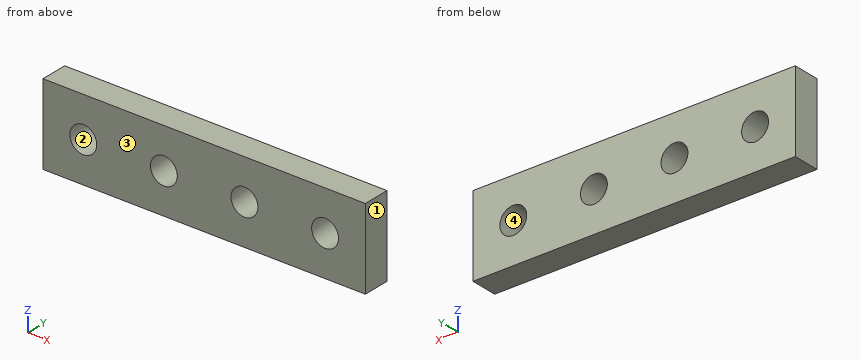
```python
from build123d import *

# Parameters (mm, degrees)
SKETCH1_W            = 120
SKETCH1_H            = 30
BOSS_EXTRUDE1_DEPTH  = 10
SKETCH2_R            = 5
CUT_EXTRUDE1_DEPTH   = 11
LPATTERN1_COUNT      = 4
LPATTERN1_PITCH      = 30
LPATTERN1_COUNT_DIR2 = 4
LPATTERN1_PITCH_DIR2 = 30


with BuildPart() as part:
    # Sketch1 → Boss-Extrude1 (new body)
    with BuildSketch(Plane(origin=(0, 0, 0), x_dir=(1, 0, 0), z_dir=(0, 1, 0))):
        with Locations((60, 15)):
            Rectangle(SKETCH1_W, SKETCH1_H)
    extrude(amount=BOSS_EXTRUDE1_DEPTH)

    # Sketch2 → Cut-Extrude1 (cut, through all)
    with BuildSketch(Plane(origin=(0, 10, 0), x_dir=(1, 0, 0), z_dir=(0, 1, 0))):
        with Locations((15, 15)):
            Circle(SKETCH2_R)
    cut_extrude1 = extrude(amount=-CUT_EXTRUDE1_DEPTH, mode=Mode.SUBTRACT)

    # LPattern1: Cut-Extrude1 4 × 4
    with Locations(*[(i * LPATTERN1_PITCH, 0, j * LPATTERN1_PITCH_DIR2) for i in range(LPATTERN1_COUNT) for j in range(LPATTERN1_COUNT_DIR2) if (i, j) != (0, 0)]):
        add(cut_extrude1, mode=Mode.SUBTRACT)


solid = part.part
```
CAD build for the part. Positions are in the model's coordinates, mm. Face numbers are marked on the shaded views. Coordinates: 2 decimals unless noted, no trailing zeros. Order: outer loops, then holes, each group sorted by start corner. A loop starts at its lowest first (then second) coordinate and runs counter-clockwise, first axis right, second up. Notation, with made-up numbers: (0, 66) - (14, 66) arc R23 cw to (14, 99) - close; hole circle Ø4 at (87.5, 23). An arc over 180 degrees is marked (long way). Use a Markdown table: item, result. Add a question column.
(1) Saw through at B-B (z = -15). Give the cut face in (x, y), then the cut area to 3 significant figures.
(2) Drill centre lines: line 1 along X through (y, z) = (6.75, -15); line 2 along Z through (x, y) = (15, 8); line 3 along X through (y, z) = (1.75, -14). Where is each one in solid material? Low to high. Write a range as [from, to].
(3) Saw through at D-D (x = 71.5). Give the cut face in (y, z).
(4) Saw through at C-C (y = 7.25). Give the cut face in (x, z).
(5) Saw through at A-A (x = 15). Give the cut face in (y, z).
(6) Pull direction X, two halves, no side cores. Call the marked faces 1, 2, 3 and 4: +X half, -X half, draft (parallel to the pull), parting line (faces both ways), or undercut.
Solved:
| question | item | result |
|---|---|---|
| 1 | outline | (0, 0) - (10, 0) - (10, 10) - (0, 10) - close; (20, 0) - (40, 0) - (40, 10) - (20, 10) - close; (50, 0) - (70, 0) - (70, 10) - (50, 10) - close; (80, 0) - (100, 0) - (100, 10) - (80, 10) - close; (110, 0) - (120, 0) - (120, 10) - (110, 10) - close |
| 1 | area | 800 mm² |
| 2 | line 1 | x = [0, 10], [20, 40], [50, 70], [80, 100], [110, 120] |
| 2 | line 2 | z = [-30, -20], [-10, 0] |
| 2 | line 3 | x = [0, 10.1], [19.9, 40.1], [49.9, 70.1], [79.9, 100.1], [109.9, 120] |
| 3 | outline | (0, -30) - (10, -30) - (10, -18.57) - (0, -18.57) - close; (0, -11.43) - (10, -11.43) - (10, 0) - (0, 0) - close |
| 4 | outline | (0, -30) - (120, -30) - (120, 0) - (0, 0) - close; hole circle Ø10 at (15, -15); hole circle Ø10 at (45, -15); hole circle Ø10 at (75, -15); hole circle Ø10 at (105, -15) |
| 5 | outline | (0, -30) - (10, -30) - (10, -20) - (0, -20) - close; (0, -10) - (10, -10) - (10, 0) - (0, 0) - close |
| 6 | face 1 | +X half |
| 6 | face 2 | undercut |
| 6 | face 3 | draft |
| 6 | face 4 | undercut |
